The drawing under review shows one solid part. Ordinate dimensions are in mm from its lowest x, y, z. A direction names the side the tool comes from. Give positions to 0.01 mm unless a question says otherwise; leave off trailing zeros. Write each loop counter-clockwise with the first axis right and the second up, starting at its lowest first coordinate (ties: lowest second). Pieces come first, ordered by that corner, then holes. Notation, with made-up numbers: (35.25, 87.25) -> (51.25, 87.25) arc R23 cw to (51.25, 99.25) -> close; hole circle Ø7 at (76, 41). An arc over 180 degrees is marked (long way). Use CSV: the item, a comma, the result in double quotes.
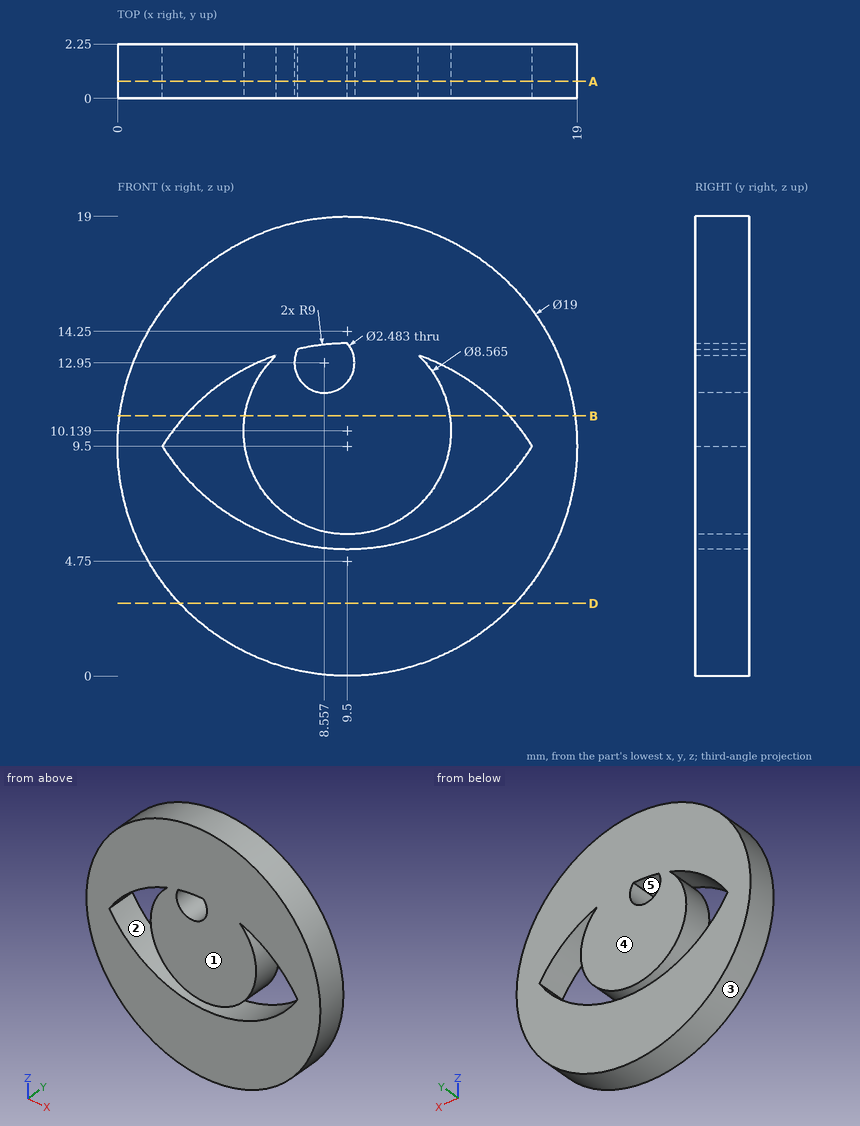
(1) Take a section at D-D (z = 3). Write out the cut boundary in (x, y).
Established:
outline,"(2.57, 0) -> (16.43, 0) -> (16.43, 2.25) -> (2.57, 2.25) -> close"
(2) For line 1 along X through (y, z) = (2, 8.25) (1 decimal); line 2 along Z through (x, y) = (8.25, 0.3); line 3 along Z through (x, y) = (6, 2.1) (1 decimal), list the stretches that pass through material, from the lowest coordinate up. Write a range as [from, to].
Established:
line 1,"x = [0.1, 2.8], [5.7, 13.3], [16.2, 18.9]"
line 2,"z = [0.08, 5.34], [6.04, 11.75], [13.66, 18.92]"
line 3,"z = [0.7, 6], [7.7, 12.6], [13, 18.3]"
(3) Tool access review of the marked faces 1 and 2: name each direction out of +Z, -Z, +X, -X, +Y, -Y from which nothing blocks a thin tool from reaching the whole face with its end or side.
Established:
face 1,"+Z, -Z, +X, -X, -Y"
face 2,"+Y, -Y"
(4) Take a section at A-A (y = 0.7). State how many separate pieces and enclosed holes the cut face has.
Established:
separate pieces,"1"
enclosed holes,"2"
(5) Mouldability with a two-part tool opening along Z and no side actions: class the marked faces 3, 4 and 5 as +Z half, -Z half, draft (parallel to the pull), parting line (faces both ways), or undercut.
Established:
face 3,"parting line"
face 4,"draft"
face 5,"undercut"
(6) Take a section at B-B (z = 10.75). Write out the cut boundary in (x, y).
Established:
outline,"(0.08, 0) -> (2.79, 0) -> (2.79, 2.25) -> (0.08, 2.25) -> close; (5.26, 0) -> (13.74, 0) -> (13.74, 2.25) -> (5.26, 2.25) -> close; (16.21, 0) -> (18.92, 0) -> (18.92, 2.25) -> (16.21, 2.25) -> close"
